from build123d import *

# Parameters (mm, degrees)
F0_R     = 33.02
F0_R_2   = 30.48
F1_DEPTH = 27.94
F3_DEPTH = 27.94
F4_DEPTH = 27.94
F6_R     = 27.305
F7_DEPTH = 25.4


with BuildPart() as f1:
    # F0 (on Front) → F1 (new body)
    with BuildSketch(Plane.XZ):
        Circle(F0_R)
        Circle(F0_R_2, mode=Mode.SUBTRACT)
    extrude(amount=F1_DEPTH)

    # F2 (on Front) → F3 (cut)
    with BuildSketch(Plane.XZ):
        with BuildLine():
            Line((-3.683, 32.8139590876), (-1.7145, 30.431741484))
            ThreePointArc((-1.7145, 30.431741484), (0, 30.48), (1.7145, 30.431741484))
            Line((1.7145, 30.431741484), (3.683, 32.8139590876))
            ThreePointArc((3.683, 32.8139590876), (0, 33.02), (-3.683, 32.8139590876))
        make_face()
        with BuildLine():
            ThreePointArc((-9.5323941009, 28.9510597855), (-7.8888044947, 29.4414191853), (-6.2202344425, 29.8385502912))
            Line((-6.2202344425, 29.8385502912), (-4.9353727389, 32.6490810886))
            ThreePointArc((-4.9353727389, 32.6490810886), (-8.5462048693, 31.8948707841), (-12.0503823753, 30.7426200024))
            Line((-12.0503823753, 30.7426200024), (-9.5323941009, 28.9510597855))
        make_face()
        with BuildLine():
            ThreePointArc((-16.7006712968, 25.4974112066), (-15.24, 26.3964543073), (-13.7310701872, 27.2119112066))
            Line((-13.7310701872, 27.2119112066), (-13.2174079816, 30.2592221686))
            ThreePointArc((-13.2174079816, 30.2592221686), (-16.51, 28.596158833), (-19.5965511059, 26.5762221686))
            Line((-19.5965511059, 26.5762221686), (-16.7006712968, 25.4974112066))
        make_face()
        with BuildLine():
            ThreePointArc((-22.730825343, 20.3061561903), (-21.5526146906, 21.5526146906), (-20.3061561903, 22.730825343))
            Line((-20.3061561903, 22.730825343), (-20.5986987133, 25.8072472635))
            ThreePointArc((-20.5986987133, 25.8072472635), (-23.3486659148, 23.3486659148), (-25.8072472635, 20.5986987133))
            Line((-25.8072472635, 20.5986987133), (-22.730825343, 20.3061561903))
        make_face()
        with BuildLine():
            ThreePointArc((-27.2119112066, 13.7310701872), (-26.3964543073, 15.24), (-25.4974112066, 16.7006712968))
            Line((-25.4974112066, 16.7006712968), (-26.5762221686, 19.5965511059))
            ThreePointArc((-26.5762221686, 19.5965511059), (-28.596158833, 16.51), (-30.2592221686, 13.2174079816))
            Line((-30.2592221686, 13.2174079816), (-27.2119112066, 13.7310701872))
        make_face()
        with BuildLine():
            ThreePointArc((-29.8385502912, 6.2202344425), (-29.4414191853, 7.8888044947), (-28.9510597855, 9.5323941009))
            Line((-28.9510597855, 9.5323941009), (-30.7426200024, 12.0503823753))
            ThreePointArc((-30.7426200024, 12.0503823753), (-31.8948707841, 8.5462048693), (-32.6490810886, 4.9353727389))
            Line((-32.6490810886, 4.9353727389), (-29.8385502912, 6.2202344425))
        make_face()
        with BuildLine():
            ThreePointArc((-30.431741484, -1.7145), (-30.48, 0), (-30.431741484, 1.7145))
            Line((-30.431741484, 1.7145), (-32.8139590876, 3.683))
            ThreePointArc((-32.8139590876, 3.683), (-33.02, 0), (-32.8139590876, -3.683))
            Line((-32.8139590876, -3.683), (-30.431741484, -1.7145))
        make_face()
        with BuildLine():
            ThreePointArc((-28.9510597855, -9.5323941009), (-29.4414191853, -7.8888044947), (-29.8385502912, -6.2202344425))
            Line((-29.8385502912, -6.2202344425), (-32.6490810886, -4.9353727389))
            ThreePointArc((-32.6490810886, -4.9353727389), (-31.8948707841, -8.5462048693), (-30.7426200024, -12.0503823753))
            Line((-30.7426200024, -12.0503823753), (-28.9510597855, -9.5323941009))
        make_face()
        with BuildLine():
            ThreePointArc((-25.4974112066, -16.7006712968), (-26.3964543073, -15.24), (-27.2119112066, -13.7310701872))
            Line((-27.2119112066, -13.7310701872), (-30.2592221686, -13.2174079816))
            ThreePointArc((-30.2592221686, -13.2174079816), (-28.596158833, -16.51), (-26.5762221686, -19.5965511059))
            Line((-26.5762221686, -19.5965511059), (-25.4974112066, -16.7006712968))
        make_face()
        with BuildLine():
            ThreePointArc((-20.3061561903, -22.730825343), (-21.5526146906, -21.5526146906), (-22.730825343, -20.3061561903))
            Line((-22.730825343, -20.3061561903), (-25.8072472635, -20.5986987133))
            ThreePointArc((-25.8072472635, -20.5986987133), (-23.3486659148, -23.3486659148), (-20.5986987133, -25.8072472635))
            Line((-20.5986987133, -25.8072472635), (-20.3061561903, -22.730825343))
        make_face()
        with BuildLine():
            ThreePointArc((-13.7310701872, -27.2119112066), (-15.24, -26.3964543073), (-16.7006712968, -25.4974112066))
            Line((-16.7006712968, -25.4974112066), (-19.5965511059, -26.5762221686))
            ThreePointArc((-19.5965511059, -26.5762221686), (-16.51, -28.596158833), (-13.2174079816, -30.2592221686))
            Line((-13.2174079816, -30.2592221686), (-13.7310701872, -27.2119112066))
        make_face()
        with BuildLine():
            ThreePointArc((-6.2202344425, -29.8385502912), (-7.8888044947, -29.4414191853), (-9.5323941009, -28.9510597855))
            Line((-9.5323941009, -28.9510597855), (-12.0503823753, -30.7426200024))
            ThreePointArc((-12.0503823753, -30.7426200024), (-8.5462048693, -31.8948707841), (-4.9353727389, -32.6490810886))
            Line((-4.9353727389, -32.6490810886), (-6.2202344425, -29.8385502912))
        make_face()
        with BuildLine():
            ThreePointArc((1.7145, -30.431741484), (0, -30.48), (-1.7145, -30.431741484))
            Line((-1.7145, -30.431741484), (-3.683, -32.8139590876))
            ThreePointArc((-3.683, -32.8139590876), (0, -33.02), (3.683, -32.8139590876))
            Line((3.683, -32.8139590876), (1.7145, -30.431741484))
        make_face()
        with BuildLine():
            ThreePointArc((9.5323941009, -28.9510597855), (7.8888044947, -29.4414191853), (6.2202344425, -29.8385502912))
            Line((6.2202344425, -29.8385502912), (4.9353727389, -32.6490810886))
            ThreePointArc((4.9353727389, -32.6490810886), (8.5462048693, -31.8948707841), (12.0503823753, -30.7426200024))
            Line((12.0503823753, -30.7426200024), (9.5323941009, -28.9510597855))
        make_face()
        with BuildLine():
            ThreePointArc((16.7006712968, -25.4974112066), (15.24, -26.3964543073), (13.7310701872, -27.2119112066))
            Line((13.7310701872, -27.2119112066), (13.2174079816, -30.2592221686))
            ThreePointArc((13.2174079816, -30.2592221686), (16.51, -28.596158833), (19.5965511059, -26.5762221686))
            Line((19.5965511059, -26.5762221686), (16.7006712968, -25.4974112066))
        make_face()
        with BuildLine():
            ThreePointArc((22.730825343, -20.3061561903), (21.5526146906, -21.5526146906), (20.3061561903, -22.730825343))
            Line((20.3061561903, -22.730825343), (20.5986987133, -25.8072472635))
            ThreePointArc((20.5986987133, -25.8072472635), (23.3486659148, -23.3486659148), (25.8072472635, -20.5986987133))
            Line((25.8072472635, -20.5986987133), (22.730825343, -20.3061561903))
        make_face()
        with BuildLine():
            ThreePointArc((27.2119112066, -13.7310701872), (26.3964543074, -15.24), (25.4974112066, -16.7006712968))
            Line((25.4974112066, -16.7006712968), (26.5762221686, -19.5965511059))
            ThreePointArc((26.5762221686, -19.5965511059), (28.596158833, -16.51), (30.2592221686, -13.2174079816))
            Line((30.2592221686, -13.2174079816), (27.2119112066, -13.7310701872))
        make_face()
        with BuildLine():
            ThreePointArc((29.8385502912, -6.2202344425), (29.4414191853, -7.8888044947), (28.9510597855, -9.5323941009))
            Line((28.9510597855, -9.5323941009), (30.7426200024, -12.0503823753))
            ThreePointArc((30.7426200024, -12.0503823753), (31.8948707841, -8.5462048693), (32.6490810886, -4.9353727389))
            Line((32.6490810886, -4.9353727389), (29.8385502912, -6.2202344425))
        make_face()
        with BuildLine():
            ThreePointArc((30.431741484, 1.7145), (30.48, 0), (30.431741484, -1.7145))
            Line((30.431741484, -1.7145), (32.8139590876, -3.683))
            ThreePointArc((32.8139590876, -3.683), (33.02, 0), (32.8139590876, 3.683))
            Line((32.8139590876, 3.683), (30.431741484, 1.7145))
        make_face()
        with BuildLine():
            ThreePointArc((28.9510597855, 9.5323941009), (29.4414191853, 7.8888044947), (29.8385502912, 6.2202344425))
            Line((29.8385502912, 6.2202344425), (32.6490810886, 4.9353727389))
            ThreePointArc((32.6490810886, 4.9353727389), (31.8948707841, 8.5462048693), (30.7426200024, 12.0503823753))
            Line((30.7426200024, 12.0503823753), (28.9510597855, 9.5323941009))
        make_face()
        with BuildLine():
            ThreePointArc((25.4974112066, 16.7006712968), (26.3964543073, 15.24), (27.2119112066, 13.7310701872))
            Line((27.2119112066, 13.7310701872), (30.2592221686, 13.2174079816))
            ThreePointArc((30.2592221686, 13.2174079816), (28.596158833, 16.51), (26.5762221686, 19.5965511059))
            Line((26.5762221686, 19.5965511059), (25.4974112066, 16.7006712968))
        make_face()
        with BuildLine():
            ThreePointArc((20.3061561903, 22.730825343), (21.5526146906, 21.5526146906), (22.730825343, 20.3061561903))
            Line((22.730825343, 20.3061561903), (25.8072472635, 20.5986987133))
            ThreePointArc((25.8072472635, 20.5986987133), (23.3486659148, 23.3486659148), (20.5986987133, 25.8072472635))
            Line((20.5986987133, 25.8072472635), (20.3061561903, 22.730825343))
        make_face()
        with BuildLine():
            ThreePointArc((13.7310701872, 27.2119112066), (15.24, 26.3964543073), (16.7006712968, 25.4974112066))
            Line((16.7006712968, 25.4974112066), (19.5965511059, 26.5762221686))
            ThreePointArc((19.5965511059, 26.5762221686), (16.51, 28.596158833), (13.2174079816, 30.2592221686))
            Line((13.2174079816, 30.2592221686), (13.7310701872, 27.2119112066))
        make_face()
        with BuildLine():
            ThreePointArc((6.2202344425, 29.8385502912), (7.8888044947, 29.4414191853), (9.5323941009, 28.9510597855))
            Line((9.5323941009, 28.9510597855), (12.0503823753, 30.7426200024))
            ThreePointArc((12.0503823753, 30.7426200024), (8.5462048693, 31.8948707841), (4.9353727389, 32.6490810886))
            Line((4.9353727389, 32.6490810886), (6.2202344425, 29.8385502912))
        make_face()
    extrude(amount=F3_DEPTH, mode=Mode.SUBTRACT)

    # F0 (on Front) → F4 (join)
    with BuildSketch(Plane.XZ):
        Circle(F0_R_2)
        with BuildLine():
            ThreePointArc((0.97536, 3.154659549), (2.6574275832, 1.9599190391), (3.302, 0))
            ThreePointArc((3.302, 0), (2.6574275832, -1.9599190391), (0.97536, -3.154659549))
            Line((0.97536, -3.154659549), (0.97536, -4.2937106432))
            Line((0.97536, -4.2937106432), (-1.05664, -4.2937106432))
            Line((-1.05664, -4.2937106432), (-1.05664, -3.1283727256))
            ThreePointArc((-1.05664, -3.1283727256), (-3.302, 0), (-1.05664, 3.1283727256))
            Line((-1.05664, 3.1283727256), (-1.05664, 4.2937106432))
            Line((-1.05664, 4.2937106432), (0.97536, 4.2937106432))
            Line((0.97536, 4.2937106432), (0.97536, 3.154659549))
        make_face(mode=Mode.SUBTRACT)
    extrude(amount=F4_DEPTH)

    # F6 (on offset) → F7 (cut)
    with BuildSketch(Plane(origin=(0, -1.27, 0), x_dir=(-1, 0, 0), z_dir=(0, 1, 0))):
        Circle(F6_R)
    extrude(amount=-F7_DEPTH, mode=Mode.SUBTRACT)


solid = f1.part
Can you work these out from the model? Positions are in its coordinate system, mm. A direction names the side the tool comes from. Round coordinates to 2 decimals unless told otherwise and drop trailing zeros. Order: outer loops, then holes, each group sorted by start corner. A loop starts at its lowest first (then second) coordinate and runs counter-clockwise, first axis right, second up. Notation, with made-up numbers: M -6.75,-14.5 L 14.25,-14.5 A15 cw 14.25,-2.5 Z; hole C 18.5,-1 d2. An arc over 180 degrees is marked long. Use a Markdown table: item, result.
1) Imagine slicing it at C-C (z = 8). List the corners of the cut face in (x, y) for me.
Geometry says:
| item | result |
|---|---|
| outline | M -29.41,-27.94 L 29.41,-27.94 L 29.41,0 L -29.41,0 Z; hole M -26.11,-26.67 L 26.11,-26.67 L 26.11,-1.27 L -26.11,-1.27 Z |
2) If I drill on line 1 along Y through (x, z) = (-20, 2); line 2 along Z through (x, y) = (-5.5, -2.5); line 3 along X through (y, z) = (-7.5, 2), over which ranges is the centre line in solid material (lowest first)?
Geometry says:
| item | result |
|---|---|
| line 1 | y = -27.94 to -26.67, -1.27 to 0 |
| line 2 | z = -31.41 to -26.75, 26.75 to 31.41 |
| line 3 | x = -30.78 to -27.23, 27.23 to 30.78 |
3) Imagine slicing it at B-B (z = 17.5). List the corners of the cut face in (x, y) for me.
Geometry says:
| item | result |
|---|---|
| outline | M -25.8,-27.94 L 25.8,-27.94 L 25.8,0 L -25.8,0 Z; hole M -20.96,-26.67 L 20.96,-26.67 L 20.96,-1.27 L -20.96,-1.27 Z |
4) I'm going to push flat-ended pins straight in: P1, Ø0.6, axis at y = -1, z = -3.5, coming from the +X side; P2, Ø1, axis at x = 0, y = -1, coming from the +Z side; P3, Ø8, axis at x = -14.5, y = -23.5, coming from the -Z side; P4, Ø1.5, axis at x = 25, y = -19.5, coming from the -Z side. Where does each tip first touch, or does it pass through?
Geometry says:
| item | result |
|---|---|
| P1 | stops at x = 32.81 |
| P2 | stops at z = 30.48 |
| P3 | stops at z = -30.74 |
| P4 | stops at z = -20.59 |
5) Imagine slicing it at A-A (x = 0). List the corners of the cut face in (y, z) for me (3 decimals), then the cut area to 3 significant figures.
Geometry says:
| item | result |
|---|---|
| outline | M -27.94,-30.48 L 0,-30.48 L 0,-4.294 L -1.27,-4.294 L -1.27,-27.305 L -26.67,-27.305 L -26.67,-4.294 L -27.94,-4.294 Z; M -27.94,4.294 L -26.67,4.294 L -26.67,27.305 L -1.27,27.305 L -1.27,4.294 L 0,4.294 L 0,30.48 L -27.94,30.48 Z |
| area | 294 mm² |
6) On a 3-axis mill with a long thin cutter (end or side, diameter ignored), from which of +Z, -Z, +X, -X, +Y, -Y can I reach the whole of each face in a straight line? I mean faces 3 (the face through (29.435, -13.774, -7.912)), 4 (the face through (10.77, -13.77, 29.83)), 5 (the face through (5.6, -13.8, -31.2)), 6 (the face through (-6, -1.27, 0)), 7 (the face through (-26.044, -13.774, -18.169)). Say none if no direction works.
Geometry says:
| item | result |
|---|---|
| face 3 | +X, +Y, -Y |
| face 4 | +Z, +Y, -Y |
| face 5 | -Z, +Y, -Y |
| face 6 | none |
| face 7 | -X, +Y, -Y |
7) If we mould it in two halves opening along Y, with no side actions, what happens to faces 1 (the face through (-5.57, -13.77, -31.26)), 2 (the face through (-6, -26.67, 0))? For each: +Y half, -Y half, draft (parallel to the pull), parting line (faces both ways), or undercut.
Geometry says:
| item | result |
|---|---|
| face 1 | draft |
| face 2 | undercut |
